```python
from build123d import *

# Parameters (mm, degrees)
SKETCH_2_W          = 14
SKETCH_2_H          = 72
CUT_EXTRUDE_1_DEPTH = 10


with BuildPart() as part:
    # 草图1 → 旋转1 (revolve)
    with BuildSketch(Plane.XY):
        Polygon((0, 0), (-136, 0), (-136, 25), (-126, 30), (-10, 30), (-10, 36), (0, 36), align=None)
    revolve(axis=Axis((0, 0, 0), (-1, 0, 0)))

    # 草图2 → 切除-拉伸1 (cut)
    with BuildSketch(Plane(origin=(0, 0, 0), x_dir=(0, 0, -1), z_dir=(1, 0, 0))):
        with Locations((-29, 0)):
            Rectangle(SKETCH_2_W, SKETCH_2_H)
    extrude(amount=-CUT_EXTRUDE_1_DEPTH, mode=Mode.SUBTRACT)


solid = part.part
```
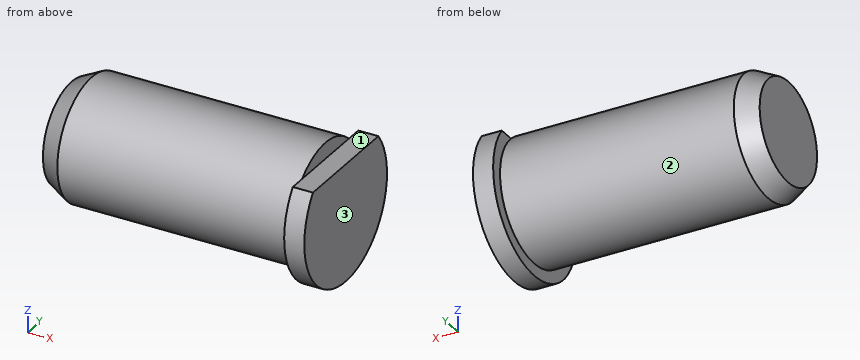
Geometry check sheet. Reference: the model listing, model coordinates, mm. Face numbers are marked on the shaded views. A direction names the side the tool comes from. Coordinates: 2 decimals unless noted, no trailing zeros. Order: outer loops, then holes, each group sorted by start corner. A loop starts at its lowest first (then second) coordinate and runs counter-clockwise, first axis right, second up.
Q1. Depth check by flat-ended pin: pin 1 Ø12 at (x, y) = (-47.5, -15.5) entering from -Z; pin 2 Ø2.5 at (y, z) = (-6.5, 24) entering from +X; pin 3 Ø4 at (y, z) = (-10, -12.5) entering from +X; pin 4 Ø5 at (x, z) = (-111.5, -23) entering from -Y. Enter the tip coordinate at first touch or a pass-through.
Reply:
pin 1: stops at z = -28.46
pin 2: stops at x = -10
pin 3: stops at x = 0
pin 4: stops at y = -21.9
Q2. Sectioned sample at A-A on y = 0. Record the cut outline in (x, z).
Reply:
outline: (-136, -25) - (-126, -30) - (-10, -30) - (-10, -36) - (0, -36) - (0, 22) - (-10, 22) - (-10, 30) - (-126, 30) - (-136, 25) - close
Q3. Tool access check on the marked faces 1, 2 and 3. Record the directions out of +Z, -Z, +X, -X, +Y, -Y that give a thin tool (end or side, any length) a straight path to the whole face; none if there is none.
Reply:
face 1: +Z, +X, +Y, -Y
face 2: -X
face 3: +Z, -Z, +X, +Y, -Y
Q4. Sectioned sample at B-B on z = 0. Record the cut outline in (x, y).
Reply:
outline: (-136, -25) - (-126, -30) - (-10, -30) - (-10, -36) - (0, -36) - (0, 36) - (-10, 36) - (-10, 30) - (-126, 30) - (-136, 25) - close
Q5. Thickness scan on probe 1 along X at (y, z) = (-32, -3.5); probe 2 along X at (y, z) = (9, 22.5); probe 3 along Y at (x, z) = (-92, -27.5). Record the ranges inside material, lowest first.
Reply:
probe 1: x = -10 to 0
probe 2: x = -136 to -10
probe 3: y = -11.99 to 11.99
Q6. Sectioned sample at C-C on x = -92. Record the cut outline in (y, z).
Reply:
outline: circle Ø60 at (0, 0)
